Geometry check sheet. Reference: the model listing, model coordinates, mm. Face numbers are marked on the shaded views. A direction names the side the tool comes from. Round coordinates to 2 decimals unless told otherwise and drop trailing zeros. Order: outer loops, then holes, each group sorted by start corner. A loop starts at its lowest first (then second) coordinate and runs counter-clockwise, first axis right, second up.
```python
from build123d import *

# Parameters (mm, degrees)
SKETCH2_R               = 7.5
BOSS_EXTRUDE1_DEPTH     = 25
CUT_EXTRUDE1_DEPTH      = 111.227038425
CUT_EXTRUDE1_DEPTH_BACK = 40
SKETCH3_W               = 30
SKETCH3_H               = 20
SKETCH4_W               = 10
SKETCH4_H               = 10
BOSS_EXTRUDE2_DEPTH     = 40
RIB36_REACH             = 112.227
SKETCH12_WALL_W         = 279.462848106
SKETCH12_WALL_H         = 10


with BuildPart() as part:
    # Sketch2 → Boss-Extrude1 (new, symmetric)
    with BuildSketch(Plane(origin=(0, 0, 0), x_dir=(0, 0, -1), z_dir=(1, 0, 0))):
        Polygon((0, 50), (40, 50), (40, 15), (95, 15), (95, 0), (0, 0), align=None)
        with Locations((20, 25)):
            Circle(SKETCH2_R, mode=Mode.SUBTRACT)
    extrude(amount=BOSS_EXTRUDE1_DEPTH, both=True)

    # Sketch3 → Cut-Extrude1 (cut, two sides: drawn at the far end of the back side and taken through both)
    with BuildSketch(Plane(origin=(0, 50, 0), x_dir=(1, 0, 0), z_dir=(0, 1, 0)).offset(-CUT_EXTRUDE1_DEPTH_BACK)):
        with Locations((0, 20)):
            Rectangle(SKETCH3_W, SKETCH3_H)
    extrude(amount=CUT_EXTRUDE1_DEPTH + CUT_EXTRUDE1_DEPTH_BACK, mode=Mode.SUBTRACT)

    # Sketch4 → Boss-Extrude2 (add)
    with BuildSketch(Plane(origin=(0, 50, 0), x_dir=(1, 0, 0), z_dir=(0, 1, 0))):
        with Locations((0, 45)):
            Rectangle(SKETCH4_W, SKETCH4_H)
    extrude(amount=-BOSS_EXTRUDE2_DEPTH)

    # Sketch12 wall → Rib36 (add, up to next)
    with BuildSketch(Plane(origin=(0, 32.5, -72.5), x_dir=(0, -0.613940613515, -0.789352217376), z_dir=(0, 0.789352217376, -0.613940613515)), mode=Mode.PRIVATE) as rib36_sk1:
        Rectangle(SKETCH12_WALL_W, SKETCH12_WALL_H)
    rib36_tool1 = extrude(rib36_sk1.sketch, amount=-RIB36_REACH, mode=Mode.PRIVATE) - part.part
    add(rib36_tool1.solids().sort_by_distance((0, 32.5, -72.5))[0])


solid = part.part
```
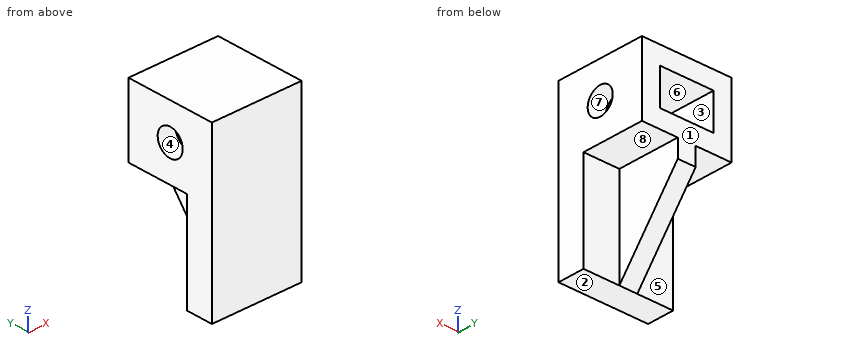
(1) Sectioned sample at D-D, the plane y = 41.5. Record the cut outline in (x, z).
Returned:
outline: (-25, -40) - (-5, -40) - (-5, -60.93) - (5, -60.93) - (5, -40) - (25, -40) - (25, 0) - (-25, 0) - close; hole (-15, -30) - (15, -30) - (15, -10) - (-15, -10) - close
(2) Sectioned sample at A-A, the plane z = -24.5. Record the cut outline in (x, y).
Returned:
outline: (-25, 0) - (25, 0) - (25, 19) - (15, 19) - (15, 10) - (-15, 10) - (-15, 19) - (-25, 19) - close; (-25, 31) - (-15, 31) - (-15, 50) - (-25, 50) - close; (15, 31) - (25, 31) - (25, 50) - (15, 50) - close
(3) Sectioned sample at C-C, the plane x = -7. Record the cut outline in (y, z), and give its area (4 significant figures).
Returned:
outline: (0, -95) - (15, -95) - (15, -40) - (50, -40) - (50, -30) - (10, -30) - (10, -10) - (50, -10) - (50, 0) - (0, 0) - close
area: 2,025 mm2
(4) Material ranges on line 1 (Z direction, x = 11, y = 32); line 2 (Y direction, x = 19.25, z = -20); line 3 (Z direction, x = -21, y = 25), recorded low to high.
Returned:
line 1: z = -40 to -30, -10 to 0
line 2: y = 0 to 17.5, 32.5 to 50
line 3: z = -40 to -27.5, -12.5 to 0
(5) Draft check along Z on the marked faces 1, 2, 3 and 4. Enter one of: released by +Z, released by -Z, zero draft, split by the parting line, or undercut.
Returned:
face 1: zero draft
face 2: released by -Z
face 3: undercut
face 4: undercut
(6) Set-up check for the marked faces 5, 6, 7 and 8: record each of +Z, -Z, +X, -X, +Y, -Y from which the full face is reachable in a straight line by a thin tool's end or side.
Returned:
face 5: -Z, -X, +Y
face 6: +Y
face 7: +X, -X
face 8: -Z, +X, +Y
(7) Sectioned sample at B-B, the plane y = 25. Record the cut outline in (x, z).
Returned:
outline: (-25, -40) - (-5, -40) - (-5, -82.14) - (5, -82.14) - (5, -40) - (25, -40) - (25, -27.5) - (15, -27.5) - (15, -30) - (-15, -30) - (-15, -27.5) - (-25, -27.5) - close; (-25, -12.5) - (-15, -12.5) - (-15, -10) - (15, -10) - (15, -12.5) - (25, -12.5) - (25, 0) - (-25, 0) - close
(8) Depth check by flat-ended pin: P1, Ø6, axis at y = 24, z = -22, coming from the +X side; P2, Ø6, axis at x = -13, z = -67.5, coming from the +Y side; P3, Ø8, axis at x = 3, z = -77.5, coming from the +Y side; P4, Ø1.5, axis at x = -14, z = -29, coming from the +Y side. Enter the tip coordinate at first touch or a pass-through.
Returned:
P1: passes through
P2: stops at y = 15
P3: stops at y = 31.72
P4: stops at y = 10
